Part model, mm, in its own coordinate system. Face numbers are marked on the shaded views. A direction names the side the tool comes from. Coordinates: 2 decimals unless noted, no trailing zeros. Write each loop counter-clockwise with the first axis right and the second up, starting at its lowest first coordinate (ties: lowest second). Pieces come first, ordered by that corner, then holes. Notation, with made-up numbers: (45.25, 52) - (64.25, 52) arc R27 cw to (64.25, 87) - close; hole circle Ø3 at (-14, 15). An arc over 180 degrees is marked (long way). Write each question's results on one line, items separated by ' | '.
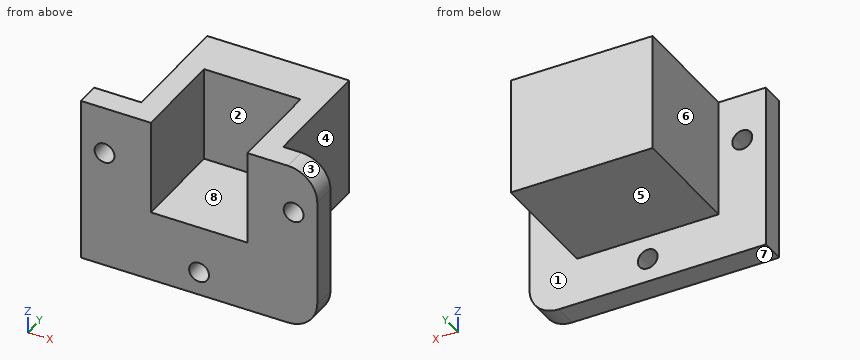
from build123d import *

# Parameters (mm, degrees)
SKETCH_1_W          = 30
SKETCH_1_H          = 30
EXTRUDE_1_DEPTH     = 5
SKETCH_2_W          = 30
SKETCH_2_H          = 5
EXTRUDE_2_DEPTH     = 10
SKETCH_3_R          = 2.1
CUT_EXTRUDE_1_DEPTH = 5
EXTRUDE_3_DEPTH     = 20
SKETCH_5_W          = 35
SKETCH_5_H          = 5
EXTRUDE_4_DEPTH     = 10
SKETCH_6_W          = 35
SKETCH_6_H          = 5
EXTRUDE_5_DEPTH     = 10
SKETCH_7_R          = 2.1
CUT_EXTRUDE_2_DEPTH = 10
FILLET_1_R          = 6.17
FILLET_2_R          = 6.17


with BuildPart() as part:
    # 스케치1 → 보스-돌출1 (new body)
    with BuildSketch(Plane.XY):
        Rectangle(SKETCH_1_W, SKETCH_1_H)
    extrude(amount=EXTRUDE_1_DEPTH)

    # 스케치2 → 보스-돌출2 (add)
    with BuildSketch(Plane(origin=(0, 0, 0), x_dir=(-1, 0, 0), z_dir=(0, 0, -1))):
        with Locations((0, -12.5)):
            Rectangle(SKETCH_2_W, SKETCH_2_H)
    extrude(amount=EXTRUDE_2_DEPTH)

    # 스케치3 → 컷-돌출1 (cut)
    with BuildSketch(Plane(origin=(0, -10, 0), x_dir=(1, 0, 0), z_dir=(0, 1, 0))):
        with Locations((0, 5)):
            Circle(SKETCH_3_R)
    extrude(amount=-CUT_EXTRUDE_1_DEPTH, mode=Mode.SUBTRACT)

    # 스케치4 → 보스-돌출3 (add)
    with BuildSketch(Plane.XY.offset(5)):
        Polygon((10.2, -15), (15, -15), (15, 15), (-15, 15), (-15, -15), (-10.2, -15), (-10.2, 5.2), (10.2, 5.2), align=None)
    extrude(amount=EXTRUDE_3_DEPTH)

    # 스케치5 → 보스-돌출4 (add)
    with BuildSketch(Plane.ZY.offset(15)):
        with Locations((7.5, -12.5)):
            Rectangle(SKETCH_5_W, SKETCH_5_H)
    extrude(amount=EXTRUDE_4_DEPTH)

    # 스케치6 → 보스-돌출5 (add)
    with BuildSketch(Plane(origin=(15, 0, 0), x_dir=(0, 0, -1), z_dir=(1, 0, 0))):
        with Locations((-7.5, -12.5)):
            Rectangle(SKETCH_6_W, SKETCH_6_H)
    extrude(amount=EXTRUDE_5_DEPTH)

    # 스케치7 → 컷-돌출2 (cut)
    with BuildSketch(Plane(origin=(0, -10, 0), x_dir=(1, 0, 0), z_dir=(0, 1, 0))):
        with Locations((-20, -15)):
            Circle(SKETCH_7_R)
        with Locations((20, -15)):
            Circle(SKETCH_7_R)
    extrude(amount=-CUT_EXTRUDE_2_DEPTH, mode=Mode.SUBTRACT)

    # 필렛1
    fillet_1_edges = [part.edges().sort_by_distance(p)[0] for p in [
        (25, -12.5, 25),
    ]]
    fillet(fillet_1_edges, radius=FILLET_1_R)

    # 필렛2
    fillet_2_edges = [part.edges().sort_by_distance(p)[0] for p in [
        (25, -12.5, -10),
    ]]
    fillet(fillet_2_edges, radius=FILLET_2_R)


solid = part.part
(1) Saw through at D-D on x = 0. Write the cut outline in (y, z), then the cut area to 3 significant figures.
Return value:
outline: (-15, -10) - (-10, -10) - (-10, -7.1) - (-15, -7.1) - close; (-15, -2.9) - (-10, -2.9) - (-10, 0) - (15, 0) - (15, 25) - (5.2, 25) - (5.2, 5) - (-15, 5) - close | area: 375 mm^2
(2) Saw through at A-A on x = -20. Write the cut outline in (y, z).
Return value:
outline: (-15, -10) - (-10, -10) - (-10, 12.9) - (-15, 12.9) - close; (-15, 17.1) - (-10, 17.1) - (-10, 25) - (-15, 25) - close
(3) Saw through at B-B on z = 15. Write the cut outline in (x, y).
Return value:
outline: (-25, -15) - (-22.1, -15) - (-22.1, -10) - (-25, -10) - close; (-17.9, -15) - (-10.2, -15) - (-10.2, 5.2) - (10.2, 5.2) - (10.2, -15) - (17.9, -15) - (17.9, -10) - (15, -10) - (15, 15) - (-15, 15) - (-15, -10) - (-17.9, -10) - close; (22.1, -15) - (25, -15) - (25, -10) - (22.1, -10) - close
(4) Wall check: line 1 (X direction, y = -11.8, z = 15); line 2 (Z direction, x = -20, y = -12.9); line 3 (X direction, y = -4.5, z = 10.5). Give the ranges that are in metal, low to high. Write a range as from..to.
Return value:
line 1: x = -25..-22.1, -17.9..-10.2, 10.2..17.9, 22.1..25 | line 2: z = -10..12.9, 17.1..25 | line 3: x = -15..-10.2, 10.2..15
(5) Two-plate mould, pull along X, no slides. Class the marked faces 1, 2 and 3: released by +X, released by -X, zero draft, split by the parting line, or undercut.
Return value:
face 1: zero draft | face 2: undercut | face 3: released by +X
(6) Saw through at C-C on y = -0.75. Write the cut outline in (x, z), then the cut area to 3 significant figures.
Return value:
outline: (-15, 0) - (15, 0) - (15, 25) - (10.2, 25) - (10.2, 5) - (-10.2, 5) - (-10.2, 25) - (-15, 25) - close | area: 342 mm^2
(7) 3-axis set-ups, long thin cutter, end or side, ignore diameter. For the marked faces 4, 5, 6, 7 and 8: which of +Z, -Z, +X, -X, +Y, -Y reach the whole face in a straight line?
Return value:
face 4: +Z, -Z, +X, +Y | face 5: -Z, +X, -X, +Y | face 6: +Z, -Z, -X, +Y | face 7: -Z, +X, -X, +Y, -Y | face 8: +Z, -Y
(8) Flat gauge pins, fed straight in: P1, Ø6, axis at x = -0.5, y = -4.5, coming from the +Z side; P2, Ø4, axis at x = 8, y = 9, coming from the -Z side; P3, Ø16, axis at x = 4, z = 19, coming from the -Y side; P4, Ø12.5, axis at y = 4, z = 9.5, coming from the +X side. Where does each tip first touch, or does it go through?
Return value:
P1: stops at z = 5 | P2: stops at z = 0 | P3: stops at y = -15 | P4: stops at x = 15
